Could you check a few things on this model? Use its own coordinates, in mm. A direction names the side the tool comes from. Coordinates: 2 decimals unless noted, no trailing zeros. Loops run counter-clockwise (first coordinate to the right, second up) from the corner with the lowest first, then second, coordinate; pieces in that order, holes last.
from build123d import *

# Parameters (mm, degrees)
SKETCH_2_R               = 4
CUT_EXTRUDE_1_DEPTH      = 20
CUT_EXTRUDE_2_DEPTH      = 10
PATTERN_CIRCULAR_1_COUNT = 17
SKETCH_4_R               = 2
CUT_EXTRUDE_3_DEPTH      = 10
SKETCH_5_R               = 2
CUT_EXTRUDE_4_DEPTH      = 10


with BuildPart() as part:
    # Sketch 1 → Revolve 1 (revolve)
    with BuildSketch(Plane.XY, mode=Mode.PRIVATE) as revolve_1_sk:
        Polygon((18, 0), (18, 9.5), (8, 9.5), (8, 7), (0, 7), (0, 0), align=None)
    revolve(revolve_1_sk.sketch.rotate(Axis((0, 0, 0), (1, 0, 0)), 90), axis=Axis((0, 0, 0), (1, 0, 0)))

    # Sketch 2 → Cut-Extrude 1 (cut)
    with BuildSketch(Plane.ZY):
        Circle(SKETCH_2_R)
    extrude(amount=-CUT_EXTRUDE_1_DEPTH, mode=Mode.SUBTRACT)

    # Sketch 3 → Cut-Extrude 2 (cut)
    with BuildSketch(Plane.ZY.offset(-8)):
        with BuildLine():
            Line((0.046298541, 7.983921855), (-0.332359624, 9.494184382))
            ThreePointArc((-0.332359624, 9.494184382), (0.866716129, 9.460380709), (2.051973159, 9.27574289))
            Line((2.051973159, 9.27574289), (1.455655646, 7.897482676))
            ThreePointArc((1.455655646, 7.897482676), (0.721917095, 7.466890324), (0.046298541, 7.983921855))
        make_face()
    cut_extrude_2 = extrude(amount=-CUT_EXTRUDE_2_DEPTH, mode=Mode.SUBTRACT)

    # Pattern Circular 1: Cut-Extrude 2 ×17 about axis
    pattern_circular_1_axis = Axis((0, 0, 0), (1, 0, 0))
    for i in range(1, PATTERN_CIRCULAR_1_COUNT):
        add(cut_extrude_2.rotate(pattern_circular_1_axis, i * 360 / PATTERN_CIRCULAR_1_COUNT), mode=Mode.SUBTRACT)

    # Sketch 4 → Cut-Extrude 3 (cut)
    with BuildSketch(Plane(origin=(0, 0, 0), x_dir=(1, 0, 0), z_dir=(0, 1, 0))):
        with Locations(Location((4, 0, 0), (0, 0, 270))):
            Circle(SKETCH_4_R)
    extrude(amount=-CUT_EXTRUDE_3_DEPTH, mode=Mode.SUBTRACT)

    # Sketch 5 → Cut-Extrude 4 (cut)
    with BuildSketch(Plane.XY):
        with Locations((4, 0)):
            Circle(SKETCH_5_R)
    extrude(amount=-CUT_EXTRUDE_4_DEPTH, mode=Mode.SUBTRACT)


solid = part.part
1) Imagine slicing it at B-B on y = 1.5. List the corners of the cut face in (x, z) for me.
2) For faces 4 (the flat face through (12.93, -8.55, 1.74)), 5 (the flat face through (12.93, 8.088, -3.284)), 6 (the flat face through (13, 8, 3)), which set-ups out of +Z, -Z, +X, -X, +Y, -Y let a thin tool reach every point of the face, with its end or its side?
3) Imagine slicing it at C-C on z = 2.5. List the corners of the cut face in (x, y) for me.
4) Will these pins go through, and if not, where does the flat tip stop? pin 1 (6.5 mm diameter, centred on x = 4, y = 0, fed in from -Z); pin 2 (5 mm diameter, centred on y = -2.5, z = 2.5, fed in from +X); pin 3 (5 mm diameter, centred on y = 0, z = 0, fed in from -X); pin 4 (10 mm diameter, centred on x = 2, y = 7.5, fed in from +Z).
5) Imagine slicing it at A-A on x = 4. List the corners of the cut face in (y, z) for me.
6) We'd pull the mould along Y, two halves only. Please class faces 1 (the cylindrical face through (12.93, 9.46, -0.89)), 2 (the flat face through (12.93, -4.043, 7.787)), 3 (the cylindrical face through (3.944, 2.681, 6.466)): released by +Y, released by -Y, zero draft, split by the parting line, or undercut.
7) If I drill on L1, parallel to X at y = -5.1, z = 0; L2, parallel to Y at x = 13.5, z = 5.5; L3, parallel to Y at x = 5.25, z = 0, over which ranges is the centre line in solid material (lowest first)?
Solved:
1. outline: (0, -6.84) - (2.68, -6.84) - (2.68, -3.71) - (0, -3.71) - close; (0, 3.71) - (18, 3.71) - (18, 9.38) - (8, 9.38) - (8, 6.84) - (0, 6.84) - close; (5.32, -6.84) - (8, -6.84) - (8, -7.36) - (18, -7.36) - (18, -3.71) - (5.32, -3.71) - close
2. face 4: +X, -X, -Y
2. face 5: +X, -X, +Y
2. face 6: +X, -X
3. outline: (0, -6.54) - (8, -6.54) - (8, -9.17) - (18, -9.17) - (18, -3.12) - (0, -3.12) - close; (0, 3.12) - (18, 3.12) - (18, 9.17) - (8, 9.17) - (8, 6.54) - (0, 6.54) - close
4. pin 1: stops at z = -7
4. pin 2: stops at x = 18
4. pin 3: passes through
4. pin 4: stops at z = 6.54
5. outline: (-6.71, -2) arc R7 ccw to (-2, -6.71) - (-2, -3.46) arc R4 cw to (-3.46, -2) - close; (-6.71, 2) - (-3.46, 2) arc R4 cw (long way) to (2, -3.46) - (2, -6.71) arc R7 ccw (long way) to start
6. face 1: released by +Y
6. face 2: undercut
6. face 3: split by the parting line
7. L1: x = 0 to 2, 6 to 18
7. L2: y = -7.75 to -6.05, -5.1 to 5.11, 6.03 to 7.75
7. L3: y = 4 to 7
